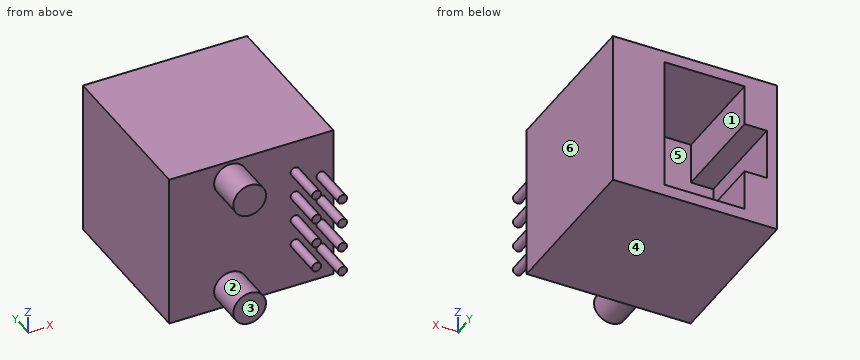
from build123d import *

# Parameters (mm, degrees)
SKETCH1_W           = 16.1
SKETCH1_H           = 16.1
BOSS_EXTRUDE1_DEPTH = 15.24
SKETCH2_R           = 1.6
BOSS_EXTRUDE2_DEPTH = 3.6
SKETCH2_4_R         = 0.45
BOSS_EXTRUDE3_DEPTH = 4
SKETCH2_5_R         = 0.45
BOSS_EXTRUDE4_DEPTH = 4
LPATTERN1_COUNT     = 3
LPATTERN1_PITCH     = 2.54
LPATTERN1_COL_COUNT = 2
LPATTERN1_COL_PITCH = 2.54
LPATTERN2_COUNT     = 2
LPATTERN2_PITCH     = 2.54
LPATTERN2_COL_COUNT = 3
LPATTERN2_COL_PITCH = 2.54
CUT_EXTRUDE1_DEPTH  = 10


with BuildPart() as part:
    # Sketch1 → Boss-Extrude1 (new body)
    with BuildSketch(Plane.XY):
        Rectangle(SKETCH1_W, SKETCH1_H)
    extrude(amount=BOSS_EXTRUDE1_DEPTH)

    # Sketch2 → Boss-Extrude2 (add)
    with BuildSketch(Plane.XZ.offset(8.05)):
        with Locations(Location((-2.05, 1.905, 0), (0, 0, 90))):
            Circle(SKETCH2_R)
        with Locations(Location((-2.05, 13.335, 0), (0, 0, 90))):
            Circle(SKETCH2_R)
    extrude(amount=BOSS_EXTRUDE2_DEPTH)

    # Sketch2_4 → Boss-Extrude3 (add)
    with BuildSketch(Plane.XZ.offset(8.05)):
        with Locations(Location((4.3, 6.985, 0), (0, 0, 90))):
            Circle(SKETCH2_4_R)
    boss_extrude3 = extrude(amount=BOSS_EXTRUDE3_DEPTH)

    # Sketch2_5 → Boss-Extrude4 (add)
    with BuildSketch(Plane.XZ.offset(8.05)):
        with Locations(Location((6.84, 8.255, 0), (0, 0, 90))):
            Circle(SKETCH2_5_R)
    boss_extrude4 = extrude(amount=BOSS_EXTRUDE4_DEPTH)

    # LPattern1: Boss-Extrude4 ×3
    with Locations(*[(0, 0, -i * LPATTERN1_PITCH) for i in range(1, LPATTERN1_COUNT)]):
        add(boss_extrude4)

    # LPattern1 col: Boss-Extrude4 ×2
    with Locations(*[(0, 0, i * LPATTERN1_COL_PITCH) for i in range(1, LPATTERN1_COL_COUNT)]):
        add(boss_extrude4)

    # LPattern2: Boss-Extrude3 ×2
    with Locations(*[(0, 0, -i * LPATTERN2_PITCH) for i in range(1, LPATTERN2_COUNT)]):
        add(boss_extrude3)

    # LPattern2 col: Boss-Extrude3 ×3
    with Locations(*[(0, 0, i * LPATTERN2_COL_PITCH) for i in range(1, LPATTERN2_COL_COUNT)]):
        add(boss_extrude3)

    # Sketch3 → Cut-Extrude1 (cut)
    with BuildSketch(Plane(origin=(0, 8.05, 0), x_dir=(1, 0, 0), z_dir=(0, 1, 0))):
        Polygon((3, -14.12), (-4.865675626, -14.12), (-4.865675626, -10.12), (-7.05, -10.12), (-7.05, -5.12), (-4.865675626, -5.12), (-4.865675626, -1.12), (3, -1.12), align=None)
    extrude(amount=-CUT_EXTRUDE1_DEPTH, mode=Mode.SUBTRACT)


solid = part.part
Can you work these out from the model? Positions are in its coordinate system, mm. Face numbers are marked on the shaded views. A direction names the side the tool comes from. Give positions to 0.01 mm unless a question says otherwise; leave off trailing zeros. Write each loop counter-clockwise with the first axis right and the second up, starting at its lowest first coordinate (ties: lowest second). Pieces come first, ordered by that corner, then holes. Notation, with made-up numbers: (-36, 4.5) -> (3, 4.5) arc R27 cw to (3, 31.5) -> close; hole circle Ø1 at (37.25, 51.5). An arc over 180 degrees is marked (long way). Answer as a JSON object with one key per item and string values. Group by question number.
Item 1: Suppose I cut it at D-D (x = 4.3). Please give me the cut outline in (y, z) (3 decimals), plus the area to 3 significant figures.
Item 2: Suppose I cut it at A-A (x = -2.05). Please give me the cut outline in (y, z) (3 decimals), plus the area to 3 significant figures.
Item 3: I'm going to push flat-ended pins straight in: P1, Ø1, axis at x = -3, z = 13, coming from the -Y side; P2, Ø0.7, axis at x = -5.5, y = 1.5, coming from the -Z side. Where does each tip first touch, or does it pass through?
Item 4: Please list where these lines run through material, in increasing order: line 1 (X direction, y = 4.5, z = 8); line 2 (X direction, y = 6, z = 12); line 3 (Y direction, x = -6.25, z = 5.75). Write a range as [from, to].
Item 5: We'd pull the mould along Z, two halves only. Please class the marked faces 4, 5 and 6: +Z half, -Z half, draft (parallel to the pull), parting line (faces both ways), or undercut.
Item 6: Suppose I cut it at B-B (y = 6.5). Please give me the cut outline in (x, z).
Item 7: Suppose I cut it at C-C (z = 13). Please give me the cut outline in (x, y), plus the area to 3 significant figures.
Item 8: For the marked faces 1, 2 and 3, which set-ups out of +Z, -Z, +X, -X, +Y, -Y let a thin tool reach every point of the face, with its end or its side?
Findings:
{
 "1": {"outline": "(-12.05, 3.995) -> (-8.05, 3.995) -> (-8.05, 0) -> (8.05, 0) -> (8.05, 15.24) -> (-8.05, 15.24) -> (-8.05, 12.515) -> (-12.05, 12.515) -> (-12.05, 11.615) -> (-8.05, 11.615) -> (-8.05, 9.975) -> (-12.05, 9.975) -> (-12.05, 9.075) -> (-8.05, 9.075) -> (-8.05, 7.435) -> (-12.05, 7.435) -> (-12.05, 6.535) -> (-8.05, 6.535) -> (-8.05, 4.895) -> (-12.05, 4.895) -> close", "area": "260 mm²"},
 "2": {"outline": "(-11.65, 0.305) -> (-8.05, 0.305) -> (-8.05, 0) -> (8.05, 0) -> (8.05, 1.12) -> (-1.95, 1.12) -> (-1.95, 14.12) -> (8.05, 14.12) -> (8.05, 15.24) -> (-8.05, 15.24) -> (-8.05, 14.935) -> (-11.65, 14.935) -> (-11.65, 11.735) -> (-8.05, 11.735) -> (-8.05, 3.505) -> (-11.65, 3.505) -> close", "area": "138 mm²"},
 "3": {"P1": "stops at y = -11.65", "P2": "stops at z = 0"},
 "4": {"line 1": "x = [-8.05, -7.05], [3, 8.05]", "line 2": "x = [-8.05, -4.87], [3, 8.05]", "line 3": "y = [-8.05, -1.95]"},
 "5": {"face 4": "-Z half", "face 5": "undercut", "face 6": "draft"},
 "6": {"outline": "(-8.05, 0) -> (8.05, 0) -> (8.05, 15.24) -> (-8.05, 15.24) -> close; hole (-7.05, 5.12) -> (-4.87, 5.12) -> (-4.87, 1.12) -> (3, 1.12) -> (3, 14.12) -> (-4.87, 14.12) -> (-4.87, 10.12) -> (-7.05, 10.12) -> close"},
 "7": {"outline": "(-8.05, -8.05) -> (-3.61, -8.05) -> (-3.61, -11.65) -> (-0.49, -11.65) -> (-0.49, -8.05) -> (8.05, -8.05) -> (8.05, 8.05) -> (3, 8.05) -> (3, -1.95) -> (-4.87, -1.95) -> (-4.87, 8.05) -> (-8.05, 8.05) -> close", "area": "192 mm²"},
 "8": {"face 1": "+Y", "face 2": "-Y", "face 3": "+Z, -Z, -X, -Y"}
}
